Could you check a few things on this model? Use its own coordinates, in mm. A direction names the side the tool comes from. Give positions to 0.01 mm unless a question says otherwise; leave off trailing zeros. Order: outer loops, then holes, each group sorted by start corner. A loop starts at its lowest first (then second) coordinate and runs counter-clockwise, first axis right, second up. Notation, with made-up numbers: (46.25, 58) -> (105.25, 58) arc R12 ccw to (105.25, 78) -> close; hole circle Ø7 at (-7.5, -35.75). An arc over 180 degrees is marked (long way). One line per item, written item: value.
```python
from build123d import *

# Parameters (mm, degrees)
SKETCH2_W               = 100
SKETCH2_H               = 100
BOSS_EXTRUDE1_DEPTH     = 10
SKETCH3_W               = 25
SKETCH3_H               = 100
BOSS_EXTRUDE2_DEPTH     = 100
CUT_EXTRUDE3_DEPTH      = 137.037678604
CUT_EXTRUDE3_DEPTH_BACK = 137.037678604
CUT_EXTRUDE4_DEPTH      = 112.411399776
CUT_EXTRUDE4_DEPTH_BACK = 112.411399776
CUT_EXTRUDE5_DEPTH      = 12
CUT_EXTRUDE7_DEPTH      = 105.910676292
CUT_EXTRUDE7_DEPTH_BACK = 10
SKETCH16_W              = 100
SKETCH16_H              = 35
SKETCH17_R              = 1.5
CUT_EXTRUDE8_DEPTH      = 105.910676292


with BuildPart() as part:
    # Sketch2 → Boss-Extrude1 (new body)
    with BuildSketch(Plane(origin=(0, 0, 0), x_dir=(1, 0, 0), z_dir=(0, 1, 0))):
        Rectangle(SKETCH2_W, SKETCH2_H)
    extrude(amount=BOSS_EXTRUDE1_DEPTH)

    # Sketch3 → Boss-Extrude2 (add)
    with BuildSketch(Plane(origin=(0, 10, 0), x_dir=(1, 0, 0), z_dir=(0, 1, 0))):
        Rectangle(SKETCH3_W, SKETCH3_H)
    extrude(amount=BOSS_EXTRUDE2_DEPTH)

    # Sketch4 → Cut-Extrude3 (cut, two sides: drawn at the far end of the back side and taken through both)
    with BuildSketch(Plane.ZY.offset(12.5).offset(-CUT_EXTRUDE3_DEPTH_BACK)):
        with BuildLine():
            ThreePointArc((5, 19.083592135), (1.769637802, 14.971315355), (0.147267966, 10))
            Line((0.147267966, 10), (50, 10))
            Line((50, 10), (50, 110))
            Line((50, 110), (-50, 110))
            Line((-50, 110), (-50, 24.347807147))
            Line((-50, 24.347807147), (5.30640787, 72.039611214))
            ThreePointArc((5.30640787, 72.039611214), (29.371344009, 75.45551054), (42.5, 55))
            ThreePointArc((42.5, 55), (35.909902577, 39.090097423), (20, 32.5))
            Line((20, 32.5), (5, 19.083592135))
        make_face()
    extrude(amount=CUT_EXTRUDE3_DEPTH + CUT_EXTRUDE3_DEPTH_BACK, mode=Mode.SUBTRACT)

    # Sketch13 → Cut-Extrude4 (cut, two sides: drawn at the far end of the back side and taken through both)
    with BuildSketch(Plane.ZY.offset(12.5).offset(-CUT_EXTRUDE4_DEPTH_BACK)):
        Polygon((3.039419763, 26.509804879), (-10.674599558, 42.413442012), (21.056943103, 69.7761758), (34.770962424, 53.872538667), align=None)
    extrude(amount=CUT_EXTRUDE4_DEPTH + CUT_EXTRUDE4_DEPTH_BACK, mode=Mode.SUBTRACT)

    # Sketch14 → Cut-Extrude5 (cut)
    with BuildSketch(Plane.ZY.offset(12.5)):
        Polygon((-15.635019711, 38.135974081), (-1.92100039, 22.232336948), (39.731382578, 58.150006598), (26.017363257, 74.053643731), align=None)
    extrude(amount=-CUT_EXTRUDE5_DEPTH, mode=Mode.SUBTRACT)

    # Sketch16 → Cut-Extrude7 (cut, two sides: drawn at the far end of the back side and taken through both)
    with BuildSketch(Plane.XZ.offset(-CUT_EXTRUDE7_DEPTH_BACK)):
        with Locations((0, 32.5)):
            Rectangle(SKETCH16_W, SKETCH16_H)
    extrude(amount=CUT_EXTRUDE7_DEPTH + CUT_EXTRUDE7_DEPTH_BACK, mode=Mode.SUBTRACT)

    # Sketch17 → Cut-Extrude8 (cut, through all)
    with BuildSketch(Plane.XZ):
        with Locations(Location((-40, 5, 0), (0, 0, 270))):
            Circle(SKETCH17_R)
        with Locations(Location((40, 5, 0), (0, 0, 270))):
            Circle(SKETCH17_R)
        with Locations(Location((40, -40, 0), (0, 0, 270))):
            Circle(SKETCH17_R)
        with Locations(Location((-40, -40, 0), (0, 0, 270))):
            Circle(SKETCH17_R)
    extrude(amount=-CUT_EXTRUDE8_DEPTH, mode=Mode.SUBTRACT)


solid = part.part
```
1) For P1, Ø12, axis at y = 55.5, z = 24, coming from the +X side; P2, Ø12, axis at x = -17, y = 59.5, coming from the -Z side; P3, Ø20.5, axis at y = 60, z = 33, coming from the -X side; P4, Ø6, axis at x = 39, z = -32.5, coming from the -Y side, each with a flat end and sliding along its axis, tell me the tip position at first contact or that it passes through.
Answer below:
P1: passes through
P2: stops at z = -13.84
P3: stops at x = -12.5
P4: stops at y = 0
2) For faces 1 (the flat face through (-1, 5, 15)), 2 (the flat face through (-6.58, 65.99, 32.97)), 3 (the flat face through (6.091, 61.936, 27.818)), 4 (the flat face through (-12.5, 43, -13)), 5 (the flat face through (0.175, 25.886, 12.605)), which set-ups out of +Z, -Z, +X, -X, +Y, -Y let a thin tool reach every point of the face, with its end or its side?
Answer below:
face 1: +Z, +X, -X, -Y
face 2: -X
face 3: +X, -X
face 4: +Z, -Z, -X, +Y
face 5: +Z, +X, -X
3) Suppose I cut it at D-D, the plane z = 17.5. Write out the boundary of the cut face in (x, y).
Answer below:
outline: (-12.5, 30.26) -> (12.5, 30.26) -> (12.5, 38.98) -> (-12.5, 38.98) -> close; (-12.5, 66.71) -> (12.5, 66.71) -> (12.5, 77.36) -> (-12.5, 77.36) -> close
4) We'd pull the mould along X, two halves only. Please class faces 6 (the flat face through (50, 5, -17)), 7 (the flat face through (6.09, 34.35, -3.72)), 8 (the flat face through (-50, 5, -17)), 9 (the cylindrical face through (-40.9, 4.9, -38.8)): +X half, -X half, draft (parallel to the pull), parting line (faces both ways), or undercut.
Answer below:
face 6: +X half
face 7: draft
face 8: -X half
face 9: undercut
5) Suppose I cut it at B-B, the plane y = 63.5. Write out the boundary of the cut face in (x, z).
Answer below:
outline: (-12.5, -4.6) -> (12.5, -4.6) -> (12.5, 13.78) -> (-12.5, 13.78) -> close; (-12.5, 35.12) -> (-0.5, 35.12) -> (-0.5, 26.47) -> (12.5, 26.47) -> (12.5, 40.83) -> (-12.5, 40.83) -> close
6) If I drill on line 1 along X through (y, z) = (2.5, 5); line 2 along X through (y, z) = (45, 27); line 3 along Y through (x, z) = (-39, -43.5), over which ranges is the centre line in solid material (lowest first)?
Answer below:
line 1: x = -50 to -41.5, -38.5 to 38.5, 41.5 to 50
line 2: x = -12.5 to 12.5
line 3: y = 0 to 10
7) Suppose I cut it at A-A, the plane x = 40. Write out the boundary of the cut face in (y, z).
Answer below:
outline: (0, -50) -> (10, -50) -> (10, -41.5) -> (0, -41.5) -> close; (0, -38.5) -> (10, -38.5) -> (10, 3.5) -> (0, 3.5) -> close; (0, 6.5) -> (10, 6.5) -> (10, 15) -> (0, 15) -> close
8) Suppose I cut it at C-C, the plane x = 4. Write out the boundary of the cut face in (y, z).
Answer below:
outline: (0, -50) -> (24.35, -50) -> (72.04, 5.31) arc R22.5 ccw (long way) to (32.5, 20) -> (19.08, 5) arc R15 cw to (10, 0.15) -> (10, 15) -> (0, 15) -> close; hole (26.51, 3.04) -> (42.41, -10.67) -> (69.78, 21.06) -> (53.87, 34.77) -> close
